Design review of the part built by this model. Coordinates are the model's own, in mm. A direction names the side the tool comes from. Coordinates: 2 decimals unless noted, no trailing zeros. Write each loop counter-clockwise with the first axis right and the second up, starting at its lowest first coordinate (ties: lowest second). Pieces come first, ordered by that corner, then holes. Notation, with made-up numbers: (-39, 21.5) - (-4, 21.5) arc R30 ccw to (-4, 43.5) - close; hole circle Ø5 at (15.5, 64.5). An arc over 180 degrees is marked (long way). Use a Markdown table: item, result.
from build123d import *

# Parameters (mm, degrees)
SKETCH1_W                = 35
SKETCH1_H                = 35
BOSS_EXTRUDE2_DEPTH      = 5
BOSS_EXTRUDE3_DEPTH      = 6
BOSS_EXTRUDE3_DEPTH_BACK = 41
SKETCH2_W                = 5
SKETCH2_H                = 3
FILLET1_R                = 1
F_3_0MM_DOWEL_HOLE1_D    = 3
SKETCH6_W                = 20
SKETCH6_H                = 3
BOSS_EXTRUDE4_DEPTH      = 20
F_5_0MM_DOWEL_HOLE1_D    = 5
FILLET2_R                = 1
FILLET3_R                = 1


with BuildPart() as part:
    # Sketch1 → Boss-Extrude2 (new body)
    with BuildSketch(Plane.XY):
        with Locations((4.15299246, 17.5)):
            Rectangle(SKETCH1_W, SKETCH1_H)
    extrude(amount=BOSS_EXTRUDE2_DEPTH)

    # Sketch2 → Boss-Extrude3 (add, two sides: drawn at the far end of the back side and taken through both)
    with BuildSketch(Plane(origin=(21.65299246, 0, 0), x_dir=(0, 0, -1), z_dir=(1, 0, 0)).offset(-BOSS_EXTRUDE3_DEPTH_BACK)):
        with Locations((-2.5, 28.5)):
            Rectangle(SKETCH2_W, SKETCH2_H)
        with Locations((-2.5, 6.5)):
            Rectangle(SKETCH2_W, SKETCH2_H)
    extrude(amount=BOSS_EXTRUDE3_DEPTH + BOSS_EXTRUDE3_DEPTH_BACK)

    # Fillet1
    fillet1_edges = [part.edges().sort_by_distance(p)[0] for p in [
        (-19.34700754, 28.5, 5),
        (-19.34700754, 28.5, 0),
        (27.65299246, 28.5, 5),
        (27.65299246, 28.5, 0),
        (-19.34700754, 6.5, 5),
        (-19.34700754, 6.5, 0),
        (27.65299246, 6.5, 5),
        (27.65299246, 6.5, 0),
    ]]
    fillet(fillet1_edges, radius=FILLET1_R)

    # Ø3.0mm Dowel Hole1 (through all)
    with Locations(Plane.XZ):
        with Locations((24.15299246, 2.5), (-15.84700754, 2.5)):
            Hole(F_3_0MM_DOWEL_HOLE1_D / 2)

    # Sketch6 → Boss-Extrude4 (add)
    with BuildSketch(Plane.XY.offset(5)):
        with Locations((4.15299246, 17.5)):
            Rectangle(SKETCH6_W, SKETCH6_H)
    extrude(amount=BOSS_EXTRUDE4_DEPTH)

    # Ø5.0mm Dowel Hole1 (through all)
    with Locations(Plane.XZ):
        with Locations((4.15299246, 15)):
            Hole(F_5_0MM_DOWEL_HOLE1_D / 2)

    # Fillet2
    fillet2_edges = [part.edges().sort_by_distance(p)[0] for p in [
        (-5.84700754, 17.5, 25),
        (14.15299246, 17.5, 25),
    ]]
    fillet(fillet2_edges, radius=FILLET2_R)

    # Fillet3
    fillet3_edges = [part.edges().sort_by_distance(p)[0] for p in [
        (21.65299246, 0, 2.5),
        (-13.34700754, 0, 2.5),
        (-13.34700754, 35, 2.5),
        (21.65299246, 35, 2.5),
    ]]
    fillet(fillet3_edges, radius=FILLET3_R)


solid = part.part
(1) Take a section at B-B on z = 15. Write out the cut boundary in (x, y).
Determined:
| item | result |
|---|---|
| outline | (-5.85, 16) - (1.65, 16) - (1.65, 19) - (-5.85, 19) - close; (6.65, 16) - (14.15, 16) - (14.15, 19) - (6.65, 19) - close |
(2) Machinability: for faces 1 (the flat face through (21.653, 32, 2)), 2 (the flat face through (-13.347, 32, 2)), 3 (the cylindrical face through (27.352, 6.521, 4.715)), 4 (the flat face through (2, 16, 17)), which of the approach directions +Z, -Z, +X, -X, +Y, -Y give a long, thin tool a straight path to every point of the face, cutting with its end or side? Answer none if there is none.
Determined:
| item | result |
|---|---|
| face 1 | +Z, -Z, +X, +Y |
| face 2 | +Z, -Z, -X, +Y |
| face 3 | +Z, +X, +Y, -Y |
| face 4 | +Z, +X, -X, -Y |
(3) Take a section at D-D on z = 2.5. State how many separate pieces and enclosed holes the cut face has, and give its area (3 significant figures).
Determined:
| item | result |
|---|---|
| separate pieces | 5 |
| enclosed holes | 0 |
| area | 1,260 mm2 |
(4) For L1, parallel to Z at x = -4, y = 29; L2, parallel to Y at x = 10, z = 7.25, list the stretches that pass through material, from the lowest coordinate up. Write a range as from..to.
Determined:
| item | result |
|---|---|
| L1 | 0..5 |
| L2 | 16..19 |
(5) For pin 1 (10 mm diameter, centred on x = 7.5, z = 13.5, fed in from -Y); pin 2 (1.2 mm diameter, centred on y = 32.5, z = 3, fed in from +X); pin 3 (2.5 mm diameter, centred on y = 14.5, z = 3.5, fed in from -X), all flat-tipped, find the tip position at first contact; note any pin that passes through.
Determined:
| item | result |
|---|---|
| pin 1 | y = 16 |
| pin 2 | x = 21.65 |
| pin 3 | x = -13.35 |
(6) Draft analysis for pull direction Y (two halves, no side actions). For faces 5 (the flat face through (26, 27, 3)), 6 (the cylindrical face through (-19.05, 28.52, 4.71)), 7 (the cylindrical face through (21.352, 34.715, 2.535)), 8 (the flat face through (26, 8, 3)), state which applies: +Y half, -Y half, draft (parallel to the pull), parting line (faces both ways), or undercut.
Determined:
| item | result |
|---|---|
| face 5 | undercut |
| face 6 | draft |
| face 7 | +Y half |
| face 8 | undercut |
(7) Take a section at A-A on y = 28. Write out the cut boundary in (x, z), and give its area (3 significant figures).
Determined:
| item | result |
|---|---|
| outline | (-19.35, 1) arc R1 ccw to (-18.35, 0) - (26.65, 0) arc R1 ccw to (27.65, 1) - (27.65, 4) arc R1 ccw to (26.65, 5) - (-18.35, 5) arc R1 ccw to (-19.35, 4) - close; hole circle Ø3 at (-15.85, 2.5); hole circle Ø3 at (24.15, 2.5) |
| area | 220 mm2 |
(8) Take a section at C-C on x = -3.5. Write out the cut boundary in (y, z).
Determined:
| item | result |
|---|---|
| outline | (0, 0) - (35, 0) - (35, 5) - (19, 5) - (19, 25) - (16, 25) - (16, 5) - (0, 5) - close |
